Could you check a few things on this model? Use its own coordinates, in mm. Face numbers are marked on the shaded views. A direction names the side the tool comes from. Coordinates: 2 decimals unless noted, no trailing zeros. Write each loop counter-clockwise with the first axis right and the second up, starting at its lowest first coordinate (ties: lowest second). Pieces come first, ordered by that corner, then holes.
Autodesk Inventor part; units mm, degrees
ref_plane "YZ Plane" through (0, 0, 0) normal (1, 0, 0) x (0, 1, 0)
ref_plane "XZ Plane" through (0, 0, 0) normal (0, 1, 0) x (-1, 0, 0)
ref_plane "XY Plane" through (0, 0, 0) normal (0, 0, 1) x (1, 0, 0)
sketch "Boceto1" plane through (0, 0, 0) normal (0, 1, 0) x (-1, 0, 0)
  line L0 (-30, -30) -> (30, -30)
  line L1 (30, -30) -> (30, 30)
  line L2 (30, 30) -> (-30, 30)
  line L3 (-30, 30) -> (-30, -30)
  line L4 (-30, -30) -> (30, 30) construction
  line L5 (30, -30) -> (-30, 30) construction
  point P0 (0, 0)
  dimension "d0" = 60
  dimension "d1" = 60
extrude "Extrusión1" add sketch "Boceto1" along normal blind 13
sketch "Boceto2" plane through (0, 13, 0) normal (0, 1, 0) x (1, 0, 0)
  circle A0 centre (0, 0) radius 27.5
  dimension "d4" = 55
extrude "Extrusión2" cut sketch "Boceto2" against normal blind 11
sketch "Boceto3" plane through (0, 2, 0) normal (0, 1, 0) x (1, 0, 0)
  circle A0 centre (0, 0) radius 27.5
hole "Agujero1" at (0, 2, 0) direction (0, -1, 0) diameter 11 depth 2
sketch "Boceto4" plane through (0, 13, 0) normal (0, 1, 0) x (1, 0, 0)
  line L0 (-30, -30) -> (30, -30)
  line L1 (30, -30) -> (30, 30)
  point P0 (0, 0)
  point P1 (25, -19)
  dimension "d14" = 11
  dimension "d15" = 5
hole "Agujero2" at (25, 13, 19) direction (0, -1, 0) diameter 4.4 end through all
pattern_linear "Patrón rectangular1" count 2 spacing 38 along (0, 0, -1) count 2 spacing 50 along (-1, 0, 0) of "Agujero2"
sketch "Boceto5" plane through (0, 2, 0) normal (0, 1, 0) x (1, 0, 0)
  circle A0 centre (0, 0) radius 24.5
  circle A1 centre (0, 0) radius 27.5
  dimension "d29" = 49
  dimension "d30" = 55
extrude "Extrusión3" add sketch "Boceto5" along normal blind 1.5
sketch "Boceto6" plane through (30, 0, 30) normal (1, 0, 0) x (0, 0, -1)
  line L0 (2.5, 13) -> (57.5, 13)
  line L1 (2.5, 13) -> (2.5, 3.5)
  line L2 (2.5, 3.5) -> (57.5, 3.5)
  line L3 (57.5, 13) -> (57.5, 3.5)
  line L4 (2.5, 13) -> (2.5, 11)
  line L5 (2.5, 11) -> (57.5, 11)
  line L6 (5.5, 3.5) -> (54.5, 3.5)
  line L7 (5.5, 3.5) -> (5.5, 11)
  circle A0 centre (5.5, 7.25) radius 3
  circle A1 centre (54.5, 7.25) radius 3
  point P0 (30, 0)
  point P1 (5.5, 7.25)
  dimension "d49" = 2
  dimension "d50" = 6
  dimension "d51" = 6
hole "Agujero3" at (30, 7.25, 24.5) at (30, 7.25, -24.5) direction (-1, 0, 0) diameter 6 depth 30
sketch "Boceto7" plane through (0, 2, 0) normal (0, 1, 0) x (1, 0, 0)
  circle A0 centre (-17.4927, -8.5006) radius 1.9922
  circle A1 centre (17.4936, -8.4925) radius 2.0099
  point P0 (0, 0)
hole "Agujero4" at (17.4936, 2, 8.4925) at (-17.4927, 2, 8.5006) direction (0, -1, 0) diameter 3 end through all countersink diameter 5.3 countersink angle 80
properties part number "Base"
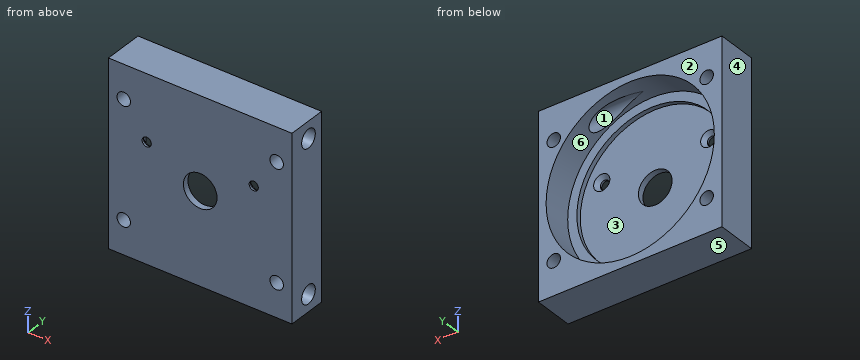
1. For pin 1 (4 mm diameter, centred on x = -25, z = 19, fed in from +Y); pin 2 (14.5 mm diameter, centred on x = 0.5, z = -1.5, fed in from +Y), each with a flat end and sliding along its axis, tell me the tip position at first contact or that it passes through.
Verdict:
pin 1: passes through
pin 2: stops at y = 2
2. I want a section at A-A on y = 5.75. Please give me the cut outline in (x, z).
Verdict:
outline: (-30, -30) - (30, -30) - (30, -27.1) - (4.68, -27.1) arc R27.5 cw (long way) to (4.68, 27.1) - (30, 27.1) - (30, 30) - (-30, 30) - close; (16.63, -21.9) - (30, -21.9) - (30, 21.9) - (16.63, 21.9) arc R27.5 cw to start; hole circle Ø4.4 at (-25, -19); hole circle Ø4.4 at (-25, 19); hole circle Ø4.4 at (25, -19); hole circle Ø4.4 at (25, 19)
3. On a 3-axis mill with a long thin cutter (end or side, diameter ignored), from which of +Z, -Z, +X, -X, +Y, -Y can I reach the whole of each face in a straight line? I mean the marked faces 1, 2 and 3. Say none if no direction works.
Verdict:
face 1: +X
face 2: +Z, -Z, +X, -X, +Y
face 3: +Y
4. If we mould it in two halves opening along X, with no side actions, what happens to the marked faces 4, 5 and 6? For each: pulls with the +X half, pulls with the -X half, needs draft (parallel to the pull), parting line crosses it, or undercut.
Verdict:
face 4: pulls with the -X half
face 5: needs draft
face 6: undercut
5. Please list where these lines run through material, in increasing order: line 1 along Z through (x, y) = (0, 10.25); line 2 along X through (y, z) = (9.25, 4).
Verdict:
line 1: z = -30 to -27.5, 27.5 to 30
line 2: x = -30 to -27.21, 27.21 to 30
6. I want a section at D-D on z = 15. Please give me the cut outline in (x, y), plus the area to 3 significant figures.
Verdict:
outline: (-30, 0) - (30, 0) - (30, 13) - (23.05, 13) - (23.05, 3.5) - (19.37, 3.5) - (19.37, 2) - (-19.37, 2) - (-19.37, 3.5) - (-23.05, 3.5) - (-23.05, 13) - (-30, 13) - close
area: 284 mm2
7. I want a section at B-B on z = 0. Please give me the cut outline in (x, y), plus the area to 3 significant figures.
Verdict:
outline: (-30, 0) - (-5.5, 0) - (-5.5, 2) - (-24.5, 2) - (-24.5, 3.5) - (-27.5, 3.5) - (-27.5, 13) - (-30, 13) - close; (5.5, 0) - (30, 0) - (30, 13) - (27.5, 13) - (27.5, 3.5) - (24.5, 3.5) - (24.5, 2) - (5.5, 2) - close
area: 162 mm2
8. I want a section at C-C on x = -9. Please give me the cut outline in (y, z), plus the area to 3 significant figures.
Verdict:
outline: (0, -30) - (13, -30) - (13, -25.99) - (3.5, -25.99) - (3.5, -22.79) - (2, -22.79) - (2, 22.79) - (3.5, 22.79) - (3.5, 25.99) - (13, 25.99) - (13, 30) - (0, 30) - close
area: 218 mm2
